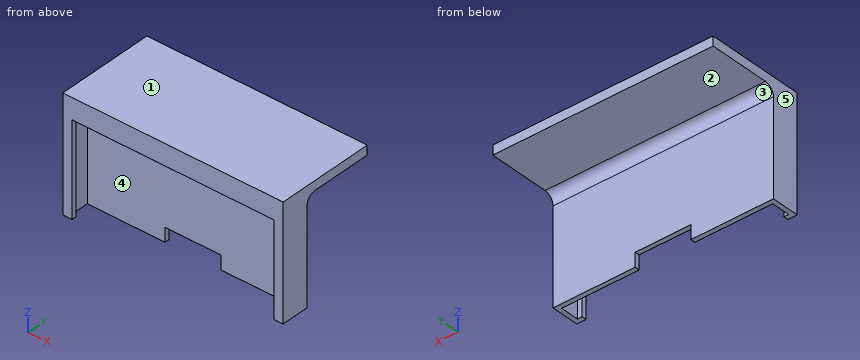
```python
from build123d import *

# Parameters (mm, degrees)
SKETCH3_W           = 47.5
SKETCH3_H           = 22.5
BOSS_EXTRUDE1_DEPTH = 6
SKETCH74_W          = 12.004185621
SKETCH74_H          = 3.004883548
CUT_EXTRUDE6_DEPTH  = 10
SKETCH79_W          = 47.5
SKETCH79_H          = 2
BOSS_EXTRUDE2_DEPTH = 21.190075336
FILLET6_R           = 2
SKETCH82_W          = 45.5
SKETCH82_H          = 4
CUT_EXTRUDE7_DEPTH  = 20.5
SKETCH84_W          = 43.5
SKETCH84_H          = 1
CUT_EXTRUDE8_DEPTH  = 20


with BuildPart() as part:
    # Sketch3 → Boss-Extrude1 (new body)
    with BuildSketch(Plane(origin=(0, 0, 0), x_dir=(1, 0, 0), z_dir=(0, 1, 0))):
        with Locations((-56.111912524, -4.514800621)):
            Rectangle(SKETCH3_W, SKETCH3_H)
    extrude(amount=BOSS_EXTRUDE1_DEPTH)

    # Sketch74 → Cut-Extrude6 (cut)
    with BuildSketch(Plane(origin=(0, 6, 0), x_dir=(1, 0, 0), z_dir=(0, 1, 0))):
        with Locations((-56.07183951, 5.232757605)):
            Rectangle(SKETCH74_W, SKETCH74_H)
    extrude(amount=-CUT_EXTRUDE6_DEPTH, mode=Mode.SUBTRACT)

    # Sketch79 → Boss-Extrude2 (add)
    with BuildSketch(Plane(origin=(0, 0, 0), x_dir=(1, 0, 0), z_dir=(0, 1, 0))):
        with Locations((-56.111912524, -16.764800621)):
            Rectangle(SKETCH79_W, SKETCH79_H)
    extrude(amount=BOSS_EXTRUDE2_DEPTH)

    # Fillet6
    fillet6_edges = [part.edges().sort_by_distance(p)[0] for p in [
        (-56.111912524, 6, 15.764800621),
    ]]
    fillet(fillet6_edges, radius=FILLET6_R)

    # Sketch82 → Cut-Extrude7 (cut)
    with BuildSketch(Plane(origin=(0, 0, -6.735199379), x_dir=(-1, 0, 0), z_dir=(0, 0, -1))):
        with Locations((56.111912524, 3)):
            Rectangle(SKETCH82_W, SKETCH82_H)
    extrude(amount=-CUT_EXTRUDE7_DEPTH, mode=Mode.SUBTRACT)

    # Sketch84 → Cut-Extrude8 (cut)
    with BuildSketch(Plane(origin=(0, 0, -6.735199379), x_dir=(-1, 0, 0), z_dir=(0, 0, -1))):
        with Locations((56.111912524, 0.5)):
            Rectangle(SKETCH84_W, SKETCH84_H)
    extrude(amount=-CUT_EXTRUDE8_DEPTH, mode=Mode.SUBTRACT)


solid = part.part
```
Could you check a few things on this model? Use its own coordinates, in mm. Face numbers are marked on the shaded views. A direction names the side the tool comes from. Round coordinates to 2 decimals unless told otherwise and drop trailing zeros. Write each loop counter-clockwise with the first axis right and the second up, starting at its lowest first coordinate (ties: lowest second). Pieces come first, ordered by that corner, then holes. Notation, with made-up numbers: M 45.5,-20.5 L 60.5,-20.5 A27 ccw 60.5,15.5 Z; hole C 16.5,42.5 d11. An arc over 180 degrees is marked long. Answer in a Markdown table with one row per item. Add a question column.
Q1. Imagine slicing it at D-D (x = -53). Please give me the cut outline in (y, z), then the cut area to 3 significant figures.
Q2. If we mould it in two halves opening along X, with no side actions, what happens to the marked faces 3, 4 and 5? For each: +X half, -X half, draft (parallel to the pull), parting line (faces both ways), or undercut.
Q3. Imagine slicing it at C-C (y = 16). Please give me the cut outline in (x, z).
Q4. Imagine slicing it at A-A (x = -36.5). Please give me the cut outline in (y, z), then the cut area to 3 significant figures.
Q5. Imagine slicing it at B-B (z = 3.5). Please give me the cut outline in (x, y).
Q6. If I drill on line 1 (X direction, y = 4.5, z = 9.5); line 2 (Z direction, x = -77, y = 10.75); line 3 (Y direction, x = -44, z = -3.5), over which ranges is the centre line in solid material (lowest first)? Write a range as from..to.
Q7. On a 3-axis mill with a long thin cutter (end or side, diameter ignored), from which of +Z, -Z, +X, -X, +Y, -Y can I reach the whole of each face in a straight line? I mean the marked faces 1 and 2. Say none if no direction works.
Q8. Will these pins go through, and if not, where does the flat tip stop? pin 1 Ø10 at (x, z) = (-48.5, -1) entering from +Y; pin 2 Ø8 at (x, y) = (-55.5, 16) entering from -Z; pin 3 Ø2 at (x, y) = (-57.5, 3.5) entering from -Z.
Values:
| question | item | result |
|---|---|---|
| 1 | outline | M 0,13.26 L 1,13.26 L 1,13.76 L 5,13.76 L 5,-3.73 L 6,-3.73 L 6,13.76 A2 cw 8,15.76 L 21.19,15.76 L 21.19,17.76 L 0,17.76 Z |
| 1 | area | 73.2 mm^2 |
| 2 | face 3 | draft |
| 2 | face 4 | undercut |
| 2 | face 5 | -X half |
| 3 | outline | M -79.86,15.76 L -32.36,15.76 L -32.36,17.76 L -79.86,17.76 Z |
| 4 | outline | M 0,13.26 L 1,13.26 L 1,13.76 L 5,13.76 L 5,-6.74 L 6,-6.74 L 6,13.76 A2 cw 8,15.76 L 21.19,15.76 L 21.19,17.76 L 0,17.76 Z |
| 4 | area | 76.2 mm^2 |
| 5 | outline | M -79.86,0 L -77.86,0 L -77.86,1 L -78.86,1 L -78.86,5 L -33.36,5 L -33.36,1 L -34.36,1 L -34.36,0 L -32.36,0 L -32.36,6 L -79.86,6 Z |
| 6 | line 1 | -79.86..-78.86, -33.36..-32.36 |
| 6 | line 2 | 15.76..17.76 |
| 6 | line 3 | 5..6 |
| 7 | face 1 | +Z, +X, -X, +Y, -Y |
| 7 | face 2 | -Z, +X, -X, +Y |
| 8 | pin 1 | y = 6 |
| 8 | pin 2 | z = 15.76 |
| 8 | pin 3 | z = 13.76 |
